Part model, mm, in its own coordinate system. A direction names the side the tool comes from. Give positions to 0.01 mm unless a question says otherwise; leave off trailing zeros. Write each loop counter-clockwise with the first axis right and the second up, starting at its lowest first coordinate (ties: lowest second). Pieces come first, ordered by that corner, then holes.
from build123d import *

# Parameters (mm, degrees)
FILLET1_R           = 0.5
CUT_EXTRUDE1_DEPTH  = 5
BOSS_EXTRUDE1_DEPTH = 5


with BuildPart() as part:
    # Sketch1 → Revolve1 (revolve)
    with BuildSketch(Plane(origin=(0, 0, 0), x_dir=(0, 0, -1), z_dir=(1, 0, 0)), mode=Mode.PRIVATE) as revolve1_sk:
        Polygon((0, 0), (0, 22.5), (-72, 22.5), (-72, 6.4), (-74.5, 6.4), (-74.5, 2.5), (-87.5, 2.5), (-87.5, 0), align=None)
    revolve(revolve1_sk.sketch.rotate(Axis((0, 0, 0), (0, 0, 1)), 90), axis=Axis((0, 0, 0), (0, 0, 1)))

    # Fillet1
    fillet1_edges = [part.edges().sort_by_distance(p)[0] for p in [
        (2.5, 0, 87.5),
        (6.4, 0, 74.5),
        (22.5, 0, 72),
        (22.5, 0, 0),
    ]]
    fillet(fillet1_edges, radius=FILLET1_R)

    # Sketch3 → Cut-Extrude1 (cut)
    with BuildSketch(Plane(origin=(22.5, 0, 0), x_dir=(0, 0, -1), z_dir=(1, 0, 0))):
        with BuildLine():
            Line((-67, -7.5), (-67, 7.5))
            Line((-67, 7.5), (-59.5, 7.5))
            ThreePointArc((-59.5, 7.5), (-52, 0), (-59.5, -7.5))
            Line((-59.5, -7.5), (-67, -7.5))
        make_face()
    cut_extrude1 = extrude(amount=-CUT_EXTRUDE1_DEPTH, mode=Mode.SUBTRACT)

    # Sketch4 → Boss-Extrude1 (add)
    with BuildSketch(Plane(origin=(17.5, 0, 0), x_dir=(0, 0, -1), z_dir=(1, 0, 0))):
        with BuildLine():
            Line((-66.5, -7), (-59.5, -7))
            ThreePointArc((-59.5, -7), (-52.5, 0), (-59.5, 7))
            Line((-59.5, 7), (-66.5, 7))
            Line((-66.5, 7), (-66.5, -7))
        make_face()
    boss_extrude1 = extrude(amount=BOSS_EXTRUDE1_DEPTH)

    # Mirror1: Cut-Extrude1, Boss-Extrude1 across plane
    add(cut_extrude1.mirror(Plane(origin=(0, 0, 0), x_dir=(0, 0, 1), z_dir=(1, 0, 0))), mode=Mode.SUBTRACT)
    add(boss_extrude1.mirror(Plane(origin=(0, 0, 0), x_dir=(0, 0, 1), z_dir=(1, 0, 0))))


solid = part.part
1) Saw through at A-A (x = 0). Write the cut outline in (y, z).
Check result:
outline: (-22.5, 0.5) arc R0.5 ccw to (-22, 0) - (22, 0) arc R0.5 ccw to (22.5, 0.5) - (22.5, 71.5) arc R0.5 ccw to (22, 72) - (6.4, 72) - (6.4, 74) arc R0.5 ccw to (5.9, 74.5) - (2.5, 74.5) - (2.5, 87) arc R0.5 ccw to (2, 87.5) - (-2, 87.5) arc R0.5 ccw to (-2.5, 87) - (-2.5, 74.5) - (-5.9, 74.5) arc R0.5 ccw to (-6.4, 74) - (-6.4, 72) - (-22, 72) arc R0.5 ccw to (-22.5, 71.5) - close
2) 3-axis set-ups, long thin cutter, end or side, ignore diameter. For faces 1 (the flat face through (-20, 0, 67)), 2 (the flat face through (-5, 5, 72)), 3 (the flat face through (0, 0, 87.5)), 4 (the flat face through (20, 0, 67)): which of +Z, -Z, +X, -X, +Y, -Y reach the whole face in a straight line?
Check result:
face 1: -X
face 2: +Z
face 3: +Z, +X, -X, +Y, -Y
face 4: +X
3) Flat gauge pins, fed straight in: P1, Ø6, axis at x = 8, z = 33.5, coming from the -Y side; P2, Ø1.5, axis at x = -21, z = 64.5, coming from the +Y side; P3, Ø5, axis at x = 8.5, y = -12.5, coming from the +Z side. Where does each tip first touch, or does it go through?
Check result:
P1: stops at y = -21.94
P2: stops at y = 9.81
P3: stops at z = 72
4) Saw through at C-C (x = -20). State how many separate pieces and enclosed holes the cut face has, and give its area (3 significant figures).
Check result:
separate pieces: 2
enclosed holes: 1
area: 1,460 mm2
5) Drill centre lines: L1, parallel to Z at x = 19.5, y = 5; L2, parallel to Z at x = 4, y = 15; L3, parallel to X at y = 7.5, z = 39. Where is each one in solid material? Low to high.
Check result:
L1: z = 0 to 53.91, 54.6 to 66.5, 67 to 72
L2: z = 0 to 72
L3: x = -21.21 to 21.21
6) Saw through at B-B (z = 42). Write the cut outline in (x, y), and give its area (3 significant figures).
Check result:
outline: circle Ø45 at (0, 0)
area: 1,590 mm2
